For this review, take the finished solid that the model builds, in its own axes (mm). A direction names the side the tool comes from. Give positions to 0.01 mm unless a question says otherwise; leave off trailing zeros. Order: outer loops, then holes, each group sorted by start corner. A loop starts at its lowest first (then second) coordinate and runs counter-clockwise, first axis right, second up.
Autodesk Inventor part; units mm, degrees
ref_plane "YZ Plane" through (0, 0, 0) normal (1, 0, 0) x (0, 1, 0)
ref_plane "XZ Plane" through (0, 0, 0) normal (0, 1, 0) x (-1, 0, 0)
ref_plane "XY Plane" through (0, 0, 0) normal (0, 0, 1) x (1, 0, 0)
sketch "Sketch1" plane through (0, 0, 0) normal (0, 1, 0) x (-1, 0, 0)
  line L0 (33.02, -8.89) -> (-33.02, -8.89)
  line L1 (-33.02, 8.89) -> (33.02, 8.89)
  arc A0 (33.02, -8.89) -> (33.02, 8.89) centre (33.02, 0) ccw
  arc A1 (-33.02, 8.89) -> (-33.02, -8.89) centre (-33.02, 0) ccw
  line L2 (41.91, -12.3525) -> (41.91, 10.1693) construction
  line L3 (-41.91, -12.3525) -> (-41.91, 10.1693) construction
  line L4 (8.89, 14.986) -> (-8.89, 14.986)
  line L5 (-8.89, 14.986) -> (-33.02, 8.89)
  line L6 (8.89, 14.986) -> (33.02, 8.89)
  point P0 (0, 0)
  dimension "d1" = 83.82
  dimension "d2" = 17.78
  dimension "d3" = 8.89
  dimension "d4" = 8.89
  dimension "d5" = 41.91
  dimension "d8" = 17.78
  dimension "d9" = 8.89
  dimension "d10" = 23.876
extrude "Extrusion1" add sketch "Sketch1" along normal blind 2.54
sketch "Sketch2" plane through (0, 2.54, 0) normal (0, 1, 0) x (1, 0, 0)
  line L0 (33.02, 8.89) -> (-33.02, 8.89)
  line L1 (-26.035, -8.89) -> (26.035, -8.89)
  line L2 (26.035, 8.89) -> (-26.035, 8.89)
  arc A0 (-26.035, 8.89) -> (-26.035, -8.89) centre (-26.035, 0) ccw
  arc A1 (26.035, -8.89) -> (26.035, 8.89) centre (26.035, 0) ccw
  line L3 (-34.925, 8.805) -> (-34.925, -8.975) construction
  line L4 (34.925, 8.805) -> (34.925, -8.975) construction
  point P0 (0, 0)
  point P1 (-26.035, 8.89)
  dimension "d11" = 69.85
  dimension "d12" = 17.78
  dimension "d13" = 8.89
  dimension "d14" = 34.925
extrude "Extrusion2" add sketch "Sketch2" along normal blind 17.78
sketch "Sketch3" plane through (0, 2.54, 0) normal (0, 1, 0) x (1, 0, 0)
  circle A0 centre (-38.4937, 0) radius 1.7526
  circle A1 centre (38.4937, 0) radius 1.7526
  line L0 (-40.2463, 0) -> (-41.91, 0) construction
  arc A2 (-33.02, 8.89) -> (-33.02, -8.89) centre (-33.02, 0) ccw
  line L1 (40.2463, 0) -> (41.91, 0) construction
  arc A3 (33.02, -8.89) -> (33.02, 8.89) centre (33.02, 0) ccw
  point P0 (0, 0)
  dimension "d18" = 3.5052
  dimension "d17" = 76.9874
extrude "Extrusion3" cut sketch "Sketch3" against normal blind 17.78
sketch "Sketch4" plane through (0, 20.32, 0) normal (0, 1, 0) x (1, 0, 0)
  line L0 (-31.75, 3.8822) -> (31.75, 3.8822)
  line L1 (31.75, 3.8822) -> (31.75, 2.6122)
  line L2 (31.75, 2.6122) -> (-31.75, 2.6122)
  line L3 (-31.75, 2.6122) -> (-31.75, 3.8822)
  line L4 (-31.75, -2.6122) -> (31.75, -2.6122)
  line L5 (31.75, -2.6122) -> (31.75, -3.8822)
  line L6 (31.75, -3.8822) -> (-31.75, -3.8822)
  line L7 (-31.75, -3.8822) -> (-31.75, -2.6122)
  line L8 (0, 0) -> (0, 2.6122) construction
  line L9 (0, 0) -> (0, -2.6122) construction
  point P0 (0, 0)
  dimension "d21" = 63.5
  dimension "d22" = 31.75
  dimension "d23" = 1.27
extrude "Extrusion4" add sketch "Sketch4" along normal blind 1.27
equation "\"d3\" = 0.5 * d2"
equation "\"d13\" = 0.5 * d12"
properties part number "Pickup"
1) Draft analysis for pull direction X (two halves, no side actions). For faces 6 (the face through (1, 0, 1)), 7 (the face through (-20.79, 1.25, 11.98)), 8 (the face through (20.79, 1.25, 11.98)), 9 (the face through (36.743, 1.288, -0.077)), state which applies: +X half, -X half, draft (parallel to the pull), parting line (faces both ways), or undercut.
Answer sheet:
face 6: draft
face 7: -X half
face 8: +X half
face 9: undercut
2) We need section D-D on z = 6.5. Give the boundary of the cut face in (x, y).
Answer sheet:
outline: (-39.08, 0) - (39.08, 0) - (39.08, 2.54) - (32.1, 2.54) - (32.1, 20.32) - (-32.1, 20.32) - (-32.1, 2.54) - (-39.08, 2.54) - close
3) Clearance check with flat-ended pins moving along their axes: pin 1 (12 mm diameter, centred on y = 3, z = 12, fed in from -X); pin 2 (4 mm diameter, centred on x = -6.5, y = 10, fed in from +Z); pin 3 (12 mm diameter, centred on x = -2.5, z = -4.5, fed in from +Y); pin 4 (1 mm diameter, centred on y = 21, z = -3, fed in from +X). State where each tip first meets the part, or that it passes through.
Answer sheet:
pin 1: stops at x = -39.56
pin 2: stops at z = 8.89
pin 3: stops at y = 21.59
pin 4: stops at x = 31.75
4) We need section A-A on z = 0. Give the boundary of the cut face in (x, y) (3 decimals), then the cut area to 3 significant figures.
Answer sheet:
outline: (-41.91, 0) - (-40.246, 0) - (-40.246, 2.54) - (-41.91, 2.54) - close; (-36.741, 0) - (36.741, 0) - (36.741, 2.54) - (34.925, 2.54) - (34.925, 20.32) - (-34.925, 20.32) - (-34.925, 2.54) - (-36.741, 2.54) - close; (40.246, 0) - (41.91, 0) - (41.91, 2.54) - (40.246, 2.54) - close
area: 1,440 mm2
5) Tool access review of faces 1 (the face through (-40.245, 1.288, -0.077)), 2 (the face through (34.923, 11.306, -0.195)), 3 (the face through (-34.923, 11.306, 0.195)), 4 (the face through (0, 11, 8.89)), 5 (the face through (0, 10, -8.89)): name each direction out of +Z, -Z, +X, -X, +Y, -Y from which nothing blocks a thin tool from reaching the whole face with its end or side.
Answer sheet:
face 1: +Y, -Y
face 2: +X, +Y
face 3: -X, +Y
face 4: +Z, +X, -X, +Y
face 5: -Z, +X, -X, +Y, -Y
6) We need section C-C on y = 18. Give the boundary of the cut face in (x, z) (3 decimals).
Answer sheet:
outline: (-26.035, -8.89) - (26.035, -8.89) arc R8.89 ccw to (26.035, 8.89) - (-26.035, 8.89) arc R8.89 ccw to start
7) To check wall thickness, follow line 1 (X direction, y = 0.95, z = 0); line 2 (Z direction, x = -18.5, y = 19); line 3 (Y direction, x = -28, z = 5.5). State the ranges of each line that lie inside material, in increasing order.
Answer sheet:
line 1: x = -41.91 to -40.25, -36.74 to 36.74, 40.25 to 41.91
line 2: z = -8.89 to 8.89
line 3: y = 0 to 20.32
8) We need section B-B on x = -4.5. Give the boundary of the cut face in (y, z).
Answer sheet:
outline: (0, -8.89) - (20.32, -8.89) - (20.32, -3.88) - (21.59, -3.88) - (21.59, -2.61) - (20.32, -2.61) - (20.32, 2.61) - (21.59, 2.61) - (21.59, 3.88) - (20.32, 3.88) - (20.32, 8.89) - (2.54, 8.89) - (2.54, 14.99) - (0, 14.99) - close
